from build123d import *

# Parameters (mm, degrees)
SKETCH1_R           = 3
SKETCH1_R_2         = 1.5
BOSS_EXTRUDE1_DEPTH = 4


with BuildPart() as part:
    # Sketch1 → Boss-Extrude1 (new body)
    with BuildSketch(Plane(origin=(0, 0, 0), x_dir=(1, 0, 0), z_dir=(0, 1, 0))):
        with BuildLine():
            Line((-4, 8.8), (-4, -6.866734973))
            ThreePointArc((-4, -6.866734973), (-4.301332982, -8.329288391), (-5.15625, -9.553617169))
            ThreePointArc((-5.15625, -9.553617169), (0, -22.5), (5.15625, -9.553617169))
            ThreePointArc((5.15625, -9.553617169), (4.301332982, -8.329288391), (4, -6.866734973))
            Line((4, -6.866734973), (4, 8.8))
            ThreePointArc((4, 8.8), (2.91629509, 11.41629509), (0.3, 12.5))
            Line((0.3, 12.5), (-0.3, 12.5))
            ThreePointArc((-0.3, 12.5), (-2.91629509, 11.41629509), (-4, 8.8))
        make_face()
        with Locations(Location((0, -15, 0), (0, 0, 270))):
            Circle(SKETCH1_R, mode=Mode.SUBTRACT)
        with Locations(Location((0, 8.5, 0), (0, 0, 270))):
            Circle(SKETCH1_R_2, mode=Mode.SUBTRACT)
        with Locations(Location((0, 4, 0), (0, 0, 270))):
            Circle(SKETCH1_R_2, mode=Mode.SUBTRACT)
    extrude(amount=BOSS_EXTRUDE1_DEPTH)


solid = part.part
The listing builds one solid part. Answer for the finished solid, in the listing's coordinates (mm). A direction names the side the tool comes from. Coordinates: 2 decimals unless noted, no trailing zeros. Write each loop counter-clockwise with the first axis right and the second up, starting at its lowest first coordinate (ties: lowest second). Pieces come first, ordered by that corner, then holes. Notation, with made-up numbers: M -10.75,5 L -4.75,5 A19 ccw -4.75,23 Z; hole C -39.75,-22.5 d3. An arc over 180 degrees is marked long. Write each question's results on one line, items separated by ' | '.
Item 1: For a pull along X with two mould halves and no side action, classify faces 4 (the face through (-0.25, 1.972, 22.496)), 5 (the face through (4.31, 1.97, 8.35)), 6 (the face through (-2.89, 1.97, -11.44)), 7 (the face through (0.45, 1.97, -2.57)) as released by +X, released by -X, zero draft, split by the parting line, or undercut.
Answer below:
face 4: split by the parting line | face 5: released by +X | face 6: released by -X | face 7: undercut
Item 2: The part is cut by section D-D on z = 5. Determine the outline of the cut face in (x, y), and give its area (3 significant figures).
Answer below:
outline: M -4,0 L 4,0 L 4,4 L -4,4 Z | area: 32.0 mm2
Item 3: The part is cut by section B-B on y = 1.9. Determine the outline of the cut face in (x, z), and give its area (3 significant figures).
Answer below:
outline: M -5.16,9.55 A3.7 cw -4,6.87 L -4,-8.8 A3.7 ccw -0.3,-12.5 L 0.3,-12.5 A3.7 ccw 4,-8.8 L 4,6.87 A3.7 cw 5.16,9.55 A7.5 ccw long Z; hole C 0,15 d6; hole C 0,-8.5 d3; hole C 0,-4 d3 | area: 292 mm2
Item 4: Consider probe 1 along X at (y, z) = (2.95, -8.5); probe 2 along X at (y, z) = (2.7, 15); probe 3 along Z at (x, y) = (-0.5, 1.85). Determine where each line is inside the solid, lowest interval first. Write a range as [from, to].
Answer below:
probe 1: [-4, -1.5], [1.5, 4] | probe 2: [-7.5, -3], [3, 7.5] | probe 3: [-12.49, -9.91], [-7.09, -5.41], [-2.59, 12.04], [17.96, 22.48]
Item 5: The part is cut by section A-A on z = 15. Determine the outline of the cut face in (x, y), and give its area (3 significant figures).
Answer below:
outline: M -7.5,0 L -3,0 L -3,4 L -7.5,4 Z; M 3,0 L 7.5,0 L 7.5,4 L 3,4 Z | area: 36.0 mm2
Item 6: The part is cut by section C-C on x = 2. Determine the outline of the cut face in (y, z), and give its area (3 significant figures).
Answer below:
outline: M 0,-12.09 L 4,-12.09 L 4,12.76 L 0,12.76 Z; M 0,17.24 L 4,17.24 L 4,22.23 L 0,22.23 Z | area: 119 mm2
Item 7: Given P1, Ø2, axis at y = 2, z = 2.5, coming from the -X side; P2, Ø1.5, axis at x = 2.5, y = 3.5, coming from the +Z side; P3, Ø1, axis at y = 2, z = 10.5, coming from the +X side, each flat-ended and moving along its own axis, determine where each tip first touches the part or whether it passes through.
Answer below:
P1: x = -4 | P2: z = 22.29 | P3: x = 6.34
Item 8: Which of the six approach directions +Z, -Z, +X, -X, +Y, -Y give full straight-line access (tool end or side, diameter ignored) to faces 1 (the face through (-4, 2, -1)), 2 (the face through (4, 2, -1)), 3 (the face through (0, 4, 5))?
Answer below:
face 1: -Z, -X, +Y, -Y | face 2: -Z, +X, +Y, -Y | face 3: +Z, -Z, +X, -X, +Y
